from build123d import *

# Parameters (mm, degrees)
F1_DEPTH = 20
F2_START = 1.5
F2_DEPTH = 17
F3_W     = 17
F3_H     = 17
F4_DEPTH = 30
F5_W     = 17
F5_H     = 17
F6_DEPTH = 30


with BuildPart() as f1:
    # F0 (on Top) → F1 (new body)
    with BuildSketch(Plane.XY):
        Polygon((8.5, -10), (10, -10), (10, 10), (-10, 10), (-10, 8.5), (-10, 0), (-10, -8.5), (-10, -10), (-8.5, -10), (0, -10), align=None)
    extrude(amount=F1_DEPTH)

    # F0 (on Top) → F2 (join)
    with BuildSketch(Plane.XY.offset(F2_START)):
        Polygon((-10, 0), (-10, 8.5), (-40, 8.5), (-40, -8.5), (-10, -8.5), align=None)
        Polygon((8.5, -40), (8.5, -10), (0, -10), (-8.5, -10), (-8.5, -40), align=None)
    extrude(amount=F2_DEPTH)

    # F3 (on face) → F4 (join)
    with BuildSketch(Plane.XY.offset(20)):
        Rectangle(F3_W, F3_H)
    extrude(amount=F4_DEPTH)

    # F5 (on face) → F6 (join)
    with BuildSketch(Plane(origin=(0, 0, 0), x_dir=(1, 0, 0), z_dir=(0, 0, -1))):
        Rectangle(F5_W, F5_H)
    extrude(amount=F6_DEPTH)


solid = f1.part
Work out the finished part from the listing and answer in its coordinate system (mm). A direction names the side the tool comes from. Give positions to 0.01 mm unless a question says otherwise; leave off trailing zeros. Order: outer loops, then holes, each group sorted by start corner. A loop starts at its lowest first (then second) coordinate and runs counter-clockwise, first axis right, second up. Notation, with made-up numbers: (65.25, 86.5) -> (101.25, 86.5) arc R19 ccw to (101.25, 109.5) -> close; hole circle Ø4 at (34.5, 14.5). An arc over 180 degrees is marked (long way). One line per item, written item: value.
Item 1: Find section B-B, the plane y = -7. Give the vertices of the cut face in (x, z).
Answer sheet:
outline: (-40, 1.5) -> (-10, 1.5) -> (-10, 0) -> (-8.5, 0) -> (-8.5, -30) -> (8.5, -30) -> (8.5, 0) -> (10, 0) -> (10, 20) -> (8.5, 20) -> (8.5, 50) -> (-8.5, 50) -> (-8.5, 20) -> (-10, 20) -> (-10, 18.5) -> (-40, 18.5) -> close
Item 2: A tool of negligible diameter and unlimited length cuts with its end or side. For faces 1 (the flat face through (8.5, 0, -15)), 2 (the flat face through (-25, -8.5, 10)), 3 (the flat face through (0, -25, 18.5)), 4 (the flat face through (-25, 0, 18.5)), 5 (the flat face through (0, -25, 1.5)), from which of +Z, -Z, +X, -X, +Y, -Y can it reach the whole face along a straight path? Write none if from no direction.
Answer sheet:
face 1: -Z, +X, +Y, -Y
face 2: +Z, -Z, -X, -Y
face 3: +Z, +X, -X, -Y
face 4: +Z, -X, +Y, -Y
face 5: -Z, +X, -X, -Y
Item 3: Find section D-D, the plane z = 27.5. Give the vertices of the cut face in (x, y).
Answer sheet:
outline: (-8.5, -8.5) -> (8.5, -8.5) -> (8.5, 8.5) -> (-8.5, 8.5) -> close
Item 4: Straight lines are drawn through the part: probe 1 along Z at (x, y) = (-11, 5); probe 2 along X at (y, z) = (5.5, 39); probe 3 along Y at (x, z) = (0.5, 1). For each, find the intervals that lie inside material, in ascending order.
Answer sheet:
probe 1: 1.5 to 18.5
probe 2: -8.5 to 8.5
probe 3: -10 to 10
Item 5: Flat-ended cylindrical pins translate along their axes: P1, Ø8.5, axis at y = -2, z = 37.5, coming from the -X side; P2, Ø2, axis at y = -32, z = 15, coming from the +X side; P3, Ø3, axis at x = 5, y = -31.5, coming from the +Z side. Find the tip coordinate at first contact, or state that the pin passes through.
Answer sheet:
P1: x = -8.5
P2: x = 8.5
P3: z = 18.5
Item 6: Find section A-A, the plane z = 10. Give the vertices of the cut face in (x, y), plus the area to 3 significant figures.
Answer sheet:
outline: (-40, -8.5) -> (-10, -8.5) -> (-10, -10) -> (-8.5, -10) -> (-8.5, -40) -> (8.5, -40) -> (8.5, -10) -> (10, -10) -> (10, 10) -> (-10, 10) -> (-10, 8.5) -> (-40, 8.5) -> close
area: 1,420 mm²
